Part model, mm, in its own coordinate system. A direction names the side the tool comes from. Coordinates: 2 decimals unless noted, no trailing zeros. Loops run counter-clockwise (first coordinate to the right, second up) from the corner with the lowest first, then second, coordinate; pieces in that order, holes last. Notation, with made-up numbers: M 8.5,49.25 L 54.5,49.25 A25 cw 54.5,74.25 Z; hole C -9,75 d8. An arc over 180 degrees is marked long. Use a Markdown table: item, result. Add a question column.
1) Band-saw the part on D-D (y = 15). List the corners of the cut face in (x, z), plus the area to 3 significant figures.
2) Pull direction X, two halves, no side cores. Call faces 6 (the flat face through (19, 18.3, 1)), 7 (the flat face through (-11.204, 12, 1)), 8 (the flat face through (-22.939, 7, 1)): released by +X, released by -X, zero draft, split by the parting line, or undercut.
3) Band-saw the part on C-C (x = 5). List the corners of the cut face in (y, z), plus the area to 3 significant figures.
4) Band-saw the part on B-B (y = 21). List the corners of the cut face in (x, z).
5) Wall check: probe 1 along X at (y, z) = (29, 15.5); probe 2 along Z at (x, y) = (-12, 24.5). Give the ranges that are in metal, low to high. Write a range as from..to.
6) Tool access for faces 1 (the flat face through (-16, 12, 0)), 2 (the flat face through (12, 12, 1.702)), 3 (the flat face through (19, 7, 1.702)), 4 (the flat face through (10.386, 12, 1)), 5 (the flat face through (-19, -4.56, 1)): list every direction of +Z, -Z, +X, -X, +Y, -Y with a clear straight run to the whole face (end or side of a thin tool).
7) Band-saw the part on A-A (z = 14.25). List the corners of the cut face in (x, y), plus the area to 3 significant figures.
8) Pin check, flat tips, straight feed: pin 1 Ø7.5 at (x, y) = (20, 5.5) entering from +Z; pin 2 Ø1.2 at (y, z) = (15.15, 10.85) entering from +X; pin 3 Ø4 at (y, z) = (4.5, 5.5) entering from +X; pin 4 Ø1 at (y, z) = (23.5, 14.5) entering from -X. Stop position of each tip, or through.
from build123d import *

# Parameters (mm, degrees)
F0_W      = 31.3436
F0_H      = 39.7764
F1_DEPTH  = 17.907
F2_W      = 27.94
F2_H      = 39.7764
F3_DEPTH  = 16.2052
F4_W      = 22.86
F4_H      = 1.7018
F5_DEPTH  = 6.858
F6_W      = 22.86
F6_H      = 1.7018
F7_DEPTH  = 6.858
F9_D      = 3.556
F11_D     = 3.1242
F13_D     = 2.0574
F14_W     = 21.59
F14_H     = 33.4264
F15_DEPTH = 25.4


with BuildPart() as f1:
    # F0 (on Top) → F1 (new body)
    with BuildSketch(Plane.XY):
        with Locations((-0.4093366692, 12.1527582612)):
            Rectangle(F0_W, F0_H)
    extrude(amount=F1_DEPTH)

    # F2 (on face) → F3 (cut)
    with BuildSketch(Plane.XY.offset(17.907)):
        with Locations((-0.4093366692, 12.1527582612)):
            Rectangle(F2_W, F2_H)
    extrude(amount=-F3_DEPTH, mode=Mode.SUBTRACT)

    # F4 (on face) → F5 (join)
    with BuildSketch(Plane(origin=(-16.0811366692, 0, 0), x_dir=(0, -1, 0), z_dir=(-1, 0, 0))):
        with Locations((-6.8695582612, 0.8509)):
            Rectangle(F4_W, F4_H)
    extrude(amount=F5_DEPTH)

    # F6 (on face) → F7 (join)
    with BuildSketch(Plane.YZ.offset(15.2624633308)):
        with Locations((6.8695582612, 0.8509)):
            Rectangle(F6_W, F6_H)
    extrude(amount=F7_DEPTH)

    # F9 (through all)
    with Locations(Plane.XY.offset(1.7018)):
        with Locations((-19.3831366692, -1.3854417388), (18.5644633308, -1.3854417388), (18.5644633308, 11.3145582612), (-19.3831366692, 11.3145582612)):
            Hole(F9_D / 2)

    # F11 (through all)
    with Locations(Plane.YZ.offset(15.2624633308)):
        with Locations((2.3483582612, 10.8966)):
            Hole(F11_D / 2)

    # F13 (through all)
    with Locations(Plane.YZ.offset(15.2624633308)):
        with Locations((15.1499590679, 10.8458)):
            Hole(F13_D / 2)

    # F14 (on face) → F15 (cut)
    with BuildSketch(Plane.XY.offset(1.7018)):
        with Locations((-0.4093366692, 12.1527582612)):
            Rectangle(F14_W, F14_H)
    extrude(amount=-F15_DEPTH, mode=Mode.SUBTRACT)


solid = f1.part
Entries:
| question | item | result |
|---|---|---|
| 1 | outline | M -22.94,0 L -11.2,0 L -11.2,1.7 L -14.38,1.7 L -14.38,9.83 L -16.08,9.83 L -16.08,1.7 L -22.94,1.7 Z; M -16.08,11.86 L -14.38,11.86 L -14.38,17.91 L -16.08,17.91 Z; M 10.39,0 L 22.12,0 L 22.12,1.7 L 15.26,1.7 L 15.26,9.83 L 13.56,9.83 L 13.56,1.7 L 10.39,1.7 Z; M 13.56,11.86 L 15.26,11.86 L 15.26,17.91 L 13.56,17.91 Z |
| 1 | area | 88.2 mm2 |
| 2 | face 6 | zero draft |
| 2 | face 7 | undercut |
| 2 | face 8 | released by -X |
| 3 | outline | M -7.74,0 L -4.56,0 L -4.56,1.7 L -7.74,1.7 Z; M 28.87,0 L 32.04,0 L 32.04,1.7 L 28.87,1.7 Z |
| 3 | area | 10.8 mm2 |
| 4 | outline | M -16.08,0 L -11.2,0 L -11.2,1.7 L -14.38,1.7 L -14.38,17.91 L -16.08,17.91 Z; M 10.39,0 L 15.26,0 L 15.26,17.91 L 13.56,17.91 L 13.56,1.7 L 10.39,1.7 Z |
| 5 | probe 1 | -16.08..-14.38, 13.56..15.26 |
| 5 | probe 2 | 0..1.7 |
| 6 | face 1 | -Z, +X, -X, +Y, -Y |
| 6 | face 2 | +Z, +Y, -Y |
| 6 | face 3 | +Z, +X, +Y, -Y |
| 6 | face 4 | +Z, -Z |
| 6 | face 5 | +Z, -Z, -X, -Y |
| 7 | outline | M -16.08,-7.74 L -14.38,-7.74 L -14.38,32.04 L -16.08,32.04 Z; M 13.56,-7.74 L 15.26,-7.74 L 15.26,32.04 L 13.56,32.04 Z |
| 7 | area | 135 mm2 |
| 8 | pin 1 | z = 1.7 |
| 8 | pin 2 | through |
| 8 | pin 3 | x = 15.26 |
| 8 | pin 4 | x = -16.08 |
